Autodesk Fusion 360 part; units mm, degrees
sketch "Sketch20" plane through (0, 0, 0) normal (0, 0, 1) x (1, 0, 0)
  line L0 (-44.25, -31.25) -> (44.25, -31.25)
  line L1 (44.25, -31.25) -> (44.25, 31.25)
  line L2 (44.25, 31.25) -> (-44.25, 31.25)
  line L3 (-44.25, 31.25) -> (-44.25, -31.25)
extrude "Extrude16" add sketch "Sketch20" along normal blind 8
fillet "Fillet3" radius 7 4 edges at (-44.25, 31.25, 4) (44.25, 31.25, 4) (44.25, -31.25, 4) (-44.25, -31.25, 4)
ref_plane "WorkPlane17" through (0, 0, 8) normal (0, 0, 1) x (1, 0, 0)
sketch "Sketch21" plane through (0, 0, 8) normal (0, 0, 1) x (1, 0, 0)
  line L0 (-34.25, -21.25) -> (34.25, -21.25)
  line L1 (34.25, -21.25) -> (34.25, 21.25)
  line L2 (34.25, 21.25) -> (-34.25, 21.25)
  line L3 (-34.25, 21.25) -> (-34.25, -21.25)
  line L4 (-31.25, -18.25) -> (31.25, -18.25)
  line L5 (31.25, -18.25) -> (31.25, 18.25)
  line L6 (31.25, 18.25) -> (-31.25, 18.25)
  line L7 (-31.25, 18.25) -> (-31.25, -18.25)
extrude "Extrude17" add sketch "Sketch21" along normal blind 30
fillet "Fillet4" radius 2.5 4 edges at (-34.25, 21.25, 23) (34.25, 21.25, 23) (34.25, -21.25, 23) (-34.25, -21.25, 23)
sketch "Sketch22" plane through (0, 0, 8) normal (0, 0, 1) x (1, 0, 0)
  line L0 (-44.25, -31.25) -> (44.25, -31.25)
  line L1 (44.25, -31.25) -> (44.25, 31.25)
  line L2 (44.25, 31.25) -> (-44.25, 31.25)
  line L3 (-44.25, 31.25) -> (-44.25, -31.25)
  line L4 (-39.25, -26.5) -> (39.25, -26.5)
  line L5 (39.25, -26.5) -> (39.25, 26.5)
  line L6 (39.25, 26.5) -> (-39.25, 26.5)
  line L7 (-39.25, 26.5) -> (-39.25, -26.5)
extrude "Extrude18" add sketch "Sketch22" along normal blind 25
sketch "Sketch23" plane through (0, 0, 8) normal (0, 0, 1) x (1, 0, 0)
  line L0 (-44.25, -31.25) -> (-39.25, -31.25)
  line L1 (-39.25, -31.25) -> (-39.25, 31.25)
  line L2 (-39.25, 31.25) -> (-44.25, 31.25)
  line L3 (-44.25, 31.25) -> (-44.25, -31.25)
extrude "Extrude19" cut sketch "Sketch23" along normal blind 25
fillet "Fillet5" radius 5 68 edges at (-33.5178, -20.5178, 8) (0, -21.25, 8) (33.5178, -20.5178, 8) (34.25, 0, 8) (33.5178, 20.5178, 8) (0, 21.25, 8) (-33.5178, 20.5178, 8) (-34.25, 0, 8) (0, -21.25, 8) (-33.5178, -20.5178, 8) (-34.25, 0, 8) (-33.5178, 20.5178, 8) (0, 21.25, 8) (33.5178, 20.5178, 8) (34.25, 0, 8) (33.5178, -20.5178, 8) (33.5178, -20.5178, 8) (34.25, 0, 8) (33.5178, 20.5178, 8) (0, 21.25, 8) (-33.5178, 20.5178, 8) (-34.25, 0, 8) (-33.5178, -20.5178, 8) (0, -21.25, 8) (33.5178, 20.5178, 8) (0, 21.25, 8) (-33.5178, 20.5178, 8) (-34.25, 0, 8) (-33.5178, -20.5178, 8) (0, -21.25, 8) (33.5178, -20.5178, 8) (34.25, 0, 8) (0, 21.25, 8) (33.5178, 20.5178, 8) (34.25, 0, 8) (33.5178, -20.5178, 8) (0, -21.25, 8) (-33.5178, -20.5178, 8) (-34.25, 0, 8) (-33.5178, 20.5178, 8) (-33.5178, 20.5178, 8) (-34.25, 0, 8) (-33.5178, -20.5178, 8) (0, -21.25, 8) (33.5178, -20.5178, 8) (34.25, 0, 8) (33.5178, 20.5178, 8) (0, 21.25, 8) (-34.25, 0, 8) (-33.5178, 20.5178, 8) (0, 21.25, 8) (33.5178, 20.5178, 8) (34.25, 0, 8) (33.5178, -20.5178, 8) (0, -21.25, 8) (-33.5178, -20.5178, 8) (0, -18.25, 8) (31.25, 0, 8) (0, 18.25, 8) (-31.25, 0, 8) (34.25, 0, 8) (33.5178, -20.5178, 8) (0, -21.25, 8) (-33.5178, -20.5178, 8) (-34.25, 0, 8) (-33.5178, 20.5178, 8) (0, 21.25, 8) (33.5178, 20.5178, 8)
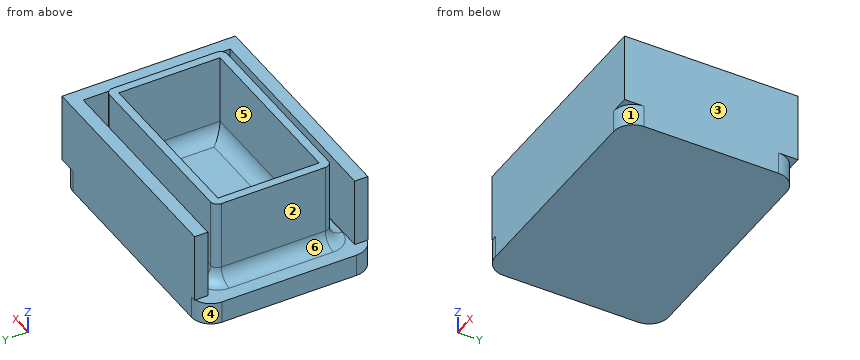
For this review, take the finished solid that the model builds, in its own axes (mm). Face numbers are marked on the shaded views. A direction names the side the tool comes from. Round coordinates to 2 decimals unless told otherwise and drop trailing zeros. Write each loop counter-clockwise with the first axis right and the second up, starting at its lowest first coordinate (ties: lowest second). Pieces come first, ordered by that corner, then holes. Notation, with made-up numbers: (6.25, -2) -> (39.25, -2) arc R13 ccw to (39.25, 4) -> close; hole circle Ø5 at (11.5, -33.5). An arc over 180 degrees is marked (long way). Put each result on its own line as item: value.
Q1. Consider section C-C on z = 35.5. State the section outline as (x, y) points.
Determined:
outline: (-34.25, -18.75) arc R2.5 ccw to (-31.75, -21.25) -> (31.75, -21.25) arc R2.5 ccw to (34.25, -18.75) -> (34.25, 18.75) arc R2.5 ccw to (31.75, 21.25) -> (-31.75, 21.25) arc R2.5 ccw to (-34.25, 18.75) -> close; hole (-31.25, -18.25) -> (31.25, -18.25) -> (31.25, 18.25) -> (-31.25, 18.25) -> close
Q2. Clearance check with flat-ended pins moving along their axes: pin 1 Ø12.5 at (y, z) = (-3, 25) entering from -X; pin 2 Ø2.5 at (y, z) = (28, 20) entering from -X; pin 3 Ø5 at (x, y) = (24, 9.5) entering from -Z; pin 4 Ø1 at (x, y) = (-31.5, -22.5) entering from +Z. State where each tip first meets the part, or that it passes through.
Determined:
pin 1: stops at x = -34.25
pin 2: stops at x = -39.25
pin 3: stops at z = 0
pin 4: stops at z = 10.37
Q3. The part is to be moulded in two halves that separate along Y. For the marked faces 1, 2 and 3, say which applies: released by +Y, released by -Y, zero draft, split by the parting line, or undercut.
Determined:
face 1: released by -Y
face 2: undercut
face 3: zero draft
Q4. Consider section A-A on z = 26.5. State the section outline as (x, y) points, and give its area (3 significant figures).
Determined:
outline: (-39.25, -31.25) -> (44.25, -31.25) -> (44.25, 31.25) -> (-39.25, 31.25) -> (-39.25, 26.5) -> (39.25, 26.5) -> (39.25, -26.5) -> (-39.25, -26.5) -> close; (-34.25, -18.75) arc R2.5 ccw to (-31.75, -21.25) -> (31.75, -21.25) arc R2.5 ccw to (34.25, -18.75) -> (34.25, 18.75) arc R2.5 ccw to (31.75, 21.25) -> (-31.75, 21.25) arc R2.5 ccw to (-34.25, 18.75) -> close; hole (-31.25, -18.25) -> (31.25, -18.25) -> (31.25, 18.25) -> (-31.25, 18.25) -> close
area: 1,680 mm^2
Q5. Consider section B-B on x = 22.5. State the section outline as (y, z) points.
Determined:
outline: (-31.25, 0) -> (31.25, 0) -> (31.25, 33) -> (26.5, 33) -> (26.5, 8) -> (26.25, 8) arc R5 cw to (21.25, 13) -> (21.25, 38) -> (18.25, 38) -> (18.25, 13) arc R5 cw to (13.25, 8) -> (-13.25, 8) arc R5 cw to (-18.25, 13) -> (-18.25, 38) -> (-21.25, 38) -> (-21.25, 13) arc R5 cw to (-26.25, 8) -> (-26.5, 8) -> (-26.5, 33) -> (-31.25, 33) -> close
Q6. Machinability: for the marked faces 4, 5 and 6, which of the approach directions +Z, -Z, +X, -X, +Y, -Y give a long, thin tool a straight path to every point of the face, cutting with its end or side? Answer none if there is none.
Determined:
face 4: -Z, -X, +Y
face 5: +Z
face 6: +Z, -X
Q7. To check wall thickness, follow L1, parallel to X at y = 1.5, z = 32; L2, parallel to Y at x = -31, z = 15; L3, parallel to Y at x = -32, z = 25. State the ranges of each line that lie inside material, in increasing order. Write a range as [from, to].
Determined:
L1: x = [-34.25, -31.25], [31.25, 34.25], [39.25, 44.25]
L2: y = [-31.25, -26.5], [-21.25, -18.25], [18.25, 21.25], [26.5, 31.25]
L3: y = [-31.25, -26.5], [-21.24, 21.24], [26.5, 31.25]
